Here's how the part is built. I have some questions about the finished solid (model axes, mm). Coordinates: 2 decimals unless noted, no trailing zeros. Write each loop counter-clockwise with the first axis right and the second up, starting at its lowest first coordinate (ties: lowest second). Pieces come first, ordered by that corner, then holes.
Item 1: If we mould it in two halves opening along Y, with no side actions, what happens to faces 1 (the face through (3, 0, -15)), 2 (the face through (3.02, 0.07, -10.5)), 3 (the face through (3, -0.9, 5.7)), 4 (the face through (3, 3, -4))? For each: pulls with the +Y half, pulls with the -Y half, needs draft (parallel to the pull), parting line crosses it, or undercut.
Item 2: I want a section at D-D (y = 1.25). Please give me the cut outline in (x, z), and give its area (4 significant figures).
Item 3: I want a section at A-A (z = 4.5). Please give me the cut outline in (x, y), and give its area (3 significant figures).
Item 4: I want a section at B-B (y = 0). Please give me the cut outline in (x, z).
Item 5: Please list where these lines run through material, in increasing order: line 1 (Y direction, x = 2.75, z = -12); line 2 (Z direction, x = 2.2, y = -0.2); line 3 (Z direction, x = 4.35, y = -0.8).
Item 6: I want a section at C-C (x = 2.6). Please give me the cut outline in (y, z).
Autodesk Inventor part; units mm, degrees
ref_plane "YZ Plane" through (0, 0, 0) normal (1, 0, 0) x (0, 1, 0)
ref_plane "XZ Plane" through (0, 0, 0) normal (0, 1, 0) x (-1, 0, 0)
ref_plane "XY Plane" through (0, 0, 0) normal (0, 0, 1) x (1, 0, 0)
sketch "Sketch1" plane through (0, 0, 0) normal (0, 0, 1) x (1, 0, 0)
  line L0 (1.5, 3) -> (4.5, 3)
  line L1 (4.5, 3) -> (4.5, -3)
  line L2 (4.5, -3) -> (1.5, -3)
  line L3 (1.5, -3) -> (1.5, 3)
  point P0 (0, 0)
extrude "Extrusion1" add sketch "Sketch1" along normal blind 8 and the other way blind 15
sketch "Sketch2" plane through (4.5, -3, 8) normal (1, 0, 0) x (0, 0, -1)
  circle A0 centre (3.5, 3) radius 1.5
  circle A1 centre (20, 3) radius 1.5
  line L0 (8, 7.2683) -> (8, -1.2683) construction
  point P0 (8, 3)
  dimension "d4" = 3
  dimension "d5" = 3
  dimension "d6" = 12
  dimension "d7" = 4.5
extrude "Extrusion2" cut sketch "Sketch2" against normal blind 8
properties part number "Bearing crossbar"
Answer:
1. face 1: needs draft
1. face 2: undercut
1. face 3: undercut
1. face 4: pulls with the +Y half
2. outline: (1.5, -15) - (4.5, -15) - (4.5, -12.83) - (1.5, -12.83) - close; (1.5, -11.17) - (4.5, -11.17) - (4.5, 3.67) - (1.5, 3.67) - close; (1.5, 5.33) - (4.5, 5.33) - (4.5, 8) - (1.5, 8) - close
2. area: 59.05 mm2
3. outline: (1.5, -3) - (4.5, -3) - (4.5, -1.5) - (1.5, -1.5) - close; (1.5, 1.5) - (4.5, 1.5) - (4.5, 3) - (1.5, 3) - close
3. area: 9.00 mm2
4. outline: (1.5, -15) - (4.5, -15) - (4.5, -13.5) - (1.5, -13.5) - close; (1.5, -10.5) - (4.5, -10.5) - (4.5, 3) - (1.5, 3) - close; (1.5, 6) - (4.5, 6) - (4.5, 8) - (1.5, 8) - close
5. line 1: y = -3 to -1.5, 1.5 to 3
5. line 2: z = -15 to -13.49, -10.51 to 3.01, 5.99 to 8
5. line 3: z = -15 to -13.27, -10.73 to 3.23, 5.77 to 8
6. outline: (-3, -15) - (3, -15) - (3, 8) - (-3, 8) - close; hole circle Ø3 at (0, -12); hole circle Ø3 at (0, 4.5)
